from build123d import *

# Parameters (mm, degrees)
F1_DEPTH = 955.675
F3_W     = 203.2
F3_H     = 152.4
F3_W_2   = 323.85
F4_DEPTH = 19.05
F6_D     = 31.75
F8_DEPTH = 19.05
F10_D    = 14.2875


with BuildPart() as f1:
    # F0 (on Right) → F1 (new body, symmetric)
    with BuildSketch(Plane.YZ):
        with BuildLine():
            Line((0, 171.45), (-355.6, 171.45))
            ThreePointArc((-355.6, 171.45), (-378.05064, 162.15064), (-387.35, 139.7))
            Line((-387.35, 139.7), (-387.35, -139.7))
            ThreePointArc((-387.35, -139.7), (-392.929616, -153.170384), (-406.4, -158.75))
            Line((-406.4, -158.75), (-514.35, -158.75))
            Line((-514.35, -158.75), (-514.35, -171.45))
            Line((-514.35, -171.45), (-406.4, -171.45))
            ThreePointArc((-406.4, -171.45), (-383.94936, -162.15064), (-374.65, -139.7))
            Line((-374.65, -139.7), (-374.65, 139.7))
            ThreePointArc((-374.65, 139.7), (-369.070384, 153.170384), (-355.6, 158.75))
            Line((-355.6, 158.75), (0, 158.75))
            Line((0, 158.75), (0, 171.45))
        make_face()
    extrude(amount=F1_DEPTH, both=True)

    # F2: F1 across plane


with BuildPart() as f1_1:
    add(f1.part)
    add(f1.part.mirror(Plane.XZ))

    # F3 (on face) → F4 (join)
    with BuildSketch(Plane.XY.offset(171.45)):
        with Locations((39.497, -266.7)):
            Rectangle(F3_W, F3_H)
        with Locations((39.497, 190.5)):
            Rectangle(F3_W, F3_H)
        with Locations((-516.128, -266.7)):
            Rectangle(F3_W_2, F3_H)
        with Locations((-516.128, 190.5)):
            Rectangle(F3_W_2, F3_H)
    extrude(amount=F4_DEPTH)

    # F6 (through all)
    with Locations(Plane.XY.offset(190.5)):
        with Locations((-582.803, 200.152), (-582.803, -276.098), (45.847, 200.152), (45.847, -276.098)):
            Hole(F6_D / 2)

    # F7 (on face) → F8 (join)
    with BuildSketch(Plane.XY.offset(171.45)):
        Polygon((-765.429, -133.35), (-765.429, -38.1), (-765.429, 57.15), (-943.229, 57.15), (-943.229, -38.1), (-943.229, -133.35), align=None)
    extrude(amount=F8_DEPTH)

    # F10 (through all)
    with Locations(Plane.XY.offset(190.5)):
        with Locations((-917.575, 28.448), (-790.575, 28.448), (-917.575, -104.902), (-790.575, -104.902)):
            Hole(F10_D / 2)


solid = f1_1.part
The listing builds one solid part. Answer for the finished solid, in the listing's coordinates (mm). A direction names the side the tool comes from. Give positions to 0.01 mm unless a question says otherwise; leave off trailing zeros. Write each loop counter-clockwise with the first axis right and the second up, starting at its lowest first coordinate (ties: lowest second). Pieces come first, ordered by that corner, then holes. Notation, with made-up numbers: (84, 44.5) -> (111, 44.5) arc R18 ccw to (111, 57.5) -> close; hole circle Ø6 at (73.25, 2). An arc over 180 degrees is marked (long way). Use a Markdown table: item, result.
(1) Find the intervals of material crossed by probe 1 along Y at (x, z) = (-332.5, 70.5); probe 2 along Z at (x, y) = (-254.5, 11); probe 3 along Y at (x, z) = (339, -140.5), in increasing order. Write a range as from..to.
Return value:
| item | result |
|---|---|
| probe 1 | -387.35..-374.65, 374.65..387.35 |
| probe 2 | 158.75..171.45 |
| probe 3 | -387.37..-374.66, 374.66..387.37 |
(2) Section C-C, the plane x = 287.5 is taken. Determine the outline of the cut face in (y, z).
Return value:
| item | result |
|---|---|
| outline | (-514.35, -171.45) -> (-406.4, -171.45) arc R31.75 ccw to (-374.65, -139.7) -> (-374.65, 139.7) arc R19.05 cw to (-355.6, 158.75) -> (355.6, 158.75) arc R19.05 cw to (374.65, 139.7) -> (374.65, -139.7) arc R31.75 ccw to (406.4, -171.45) -> (514.35, -171.45) -> (514.35, -158.75) -> (406.4, -158.75) arc R19.05 cw to (387.35, -139.7) -> (387.35, 139.7) arc R31.75 ccw to (355.6, 171.45) -> (-355.6, 171.45) arc R31.75 ccw to (-387.35, 139.7) -> (-387.35, -139.7) arc R19.05 cw to (-406.4, -158.75) -> (-514.35, -158.75) -> close |
(3) Flat-ended cylindrical pins translate along their axes: P1, Ø5, axis at x = -412.5, y = 380, coming from the -Z side; P2, Ø6, axis at x = -331.5, y = -342, coming from the +Z side; P3, Ø3, axis at x = 733.5, z = 34.5, coming from the -Y side; P4, Ø13, axis at x = -790.575, y = 28.448, coming from the +Z side. Find the tip coordinate at first contact, or state that the pin passes through.
Return value:
| item | result |
|---|---|
| P1 | z = -160.6 |
| P2 | z = 171.45 |
| P3 | y = -387.35 |
| P4 | through |
(4) Section D-D, the plane y = 153 is taken. Determine the outline of the cut face in (x, z) (3 decimals).
Return value:
| item | result |
|---|---|
| outline | (-955.675, 158.75) -> (955.675, 158.75) -> (955.675, 171.45) -> (141.097, 171.45) -> (141.097, 190.5) -> (-62.103, 190.5) -> (-62.103, 171.45) -> (-354.203, 171.45) -> (-354.203, 190.5) -> (-678.053, 190.5) -> (-678.053, 171.45) -> (-955.675, 171.45) -> close |
(5) Section A-A, the plane z = 107 is taken. Determine the outline of the cut face in (x, y) (3 decimals), then the cut area to 3 significant figures.
Return value:
| item | result |
|---|---|
| outline | (-955.675, -387.35) -> (955.675, -387.35) -> (955.675, -374.65) -> (-955.675, -374.65) -> close; (-955.675, 374.65) -> (955.675, 374.65) -> (955.675, 387.35) -> (-955.675, 387.35) -> close |
| area | 48,500 mm2 |
(6) Determine the mould class of faces 1 (the flat face through (13, -387.35, 2)), 2 (the flat face through (13, 374.65, -2)), 3 (the flat face through (13, -5, 171.45)), 4 (the flat face through (955.675, 2, 166)) for opening direction Y: released by +Y, released by -Y, zero draft, split by the parting line, or undercut.
Return value:
| item | result |
|---|---|
| face 1 | released by -Y |
| face 2 | undercut |
| face 3 | undercut |
| face 4 | zero draft |
(7) Section B-B, the plane y = -49 is taken. Determine the outline of the cut face in (x, z) (3 decimals), then the cut area to 3 significant figures.
Return value:
| item | result |
|---|---|
| outline | (-955.675, 158.75) -> (955.675, 158.75) -> (955.675, 171.45) -> (-765.429, 171.45) -> (-765.429, 190.5) -> (-943.229, 190.5) -> (-943.229, 171.45) -> (-955.675, 171.45) -> close |
| area | 27,700 mm2 |
(8) For faces 5 (the flat face through (13, 387.35, 2)), 6 (the flat face through (13, -460, -158.75)), 7 (the flat face through (-856, -37, 190.5)), 8 (the flat face through (13, 5, 158.75)), determine the directions among +Z, -Z, +X, -X, +Y, -Y from which every point of the face is accessible in a straight line to the end or side of a thin tool.
Return value:
| item | result |
|---|---|
| face 5 | +Z, +X, -X, +Y |
| face 6 | +Z, +X, -X, -Y |
| face 7 | +Z, +X, -X, +Y, -Y |
| face 8 | -Z, +X, -X |
